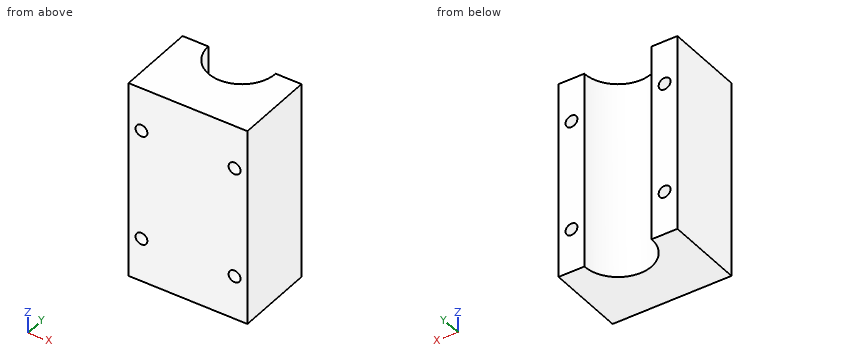
from build123d import *

# Parameters (mm, degrees)
F0_W     = 60
F0_H     = 40
F1_DEPTH = 100
F2_R     = 17
F3_DEPTH = 100
F4_R     = 3
F5_DEPTH = 45


with BuildPart() as f1:
    # F0 (on Top) → F1 (new body)
    with BuildSketch(Plane.XY):
        with Locations((0, -20)):
            Rectangle(F0_W, F0_H)
    extrude(amount=F1_DEPTH)

    # F2 (on face) → F3 (cut)
    with BuildSketch(Plane.XY.offset(100)):
        Circle(F2_R)
    extrude(amount=-F3_DEPTH, mode=Mode.SUBTRACT)

    # F4 (on face) → F5 (cut)
    with BuildSketch(Plane.XZ.offset(40)):
        with Locations((-23.5, 78)):
            Circle(F4_R)
        with Locations((-23.5, 22)):
            Circle(F4_R)
        with Locations((23.5, 22)):
            Circle(F4_R)
        with Locations((23.5, 78)):
            Circle(F4_R)
    extrude(amount=-F5_DEPTH, mode=Mode.SUBTRACT)


solid = f1.part
Could you check a few things on this model? Use its own coordinates, in mm. Give positions to 0.01 mm unless a question says otherwise; leave off trailing zeros. Order: outer loops, then holes, each group sorted by start corner. A loop starts at its lowest first (then second) coordinate and runs counter-clockwise, first axis right, second up.
Item 1: I need wall thicknesses on line 1 (Z direction, x = 23.5, y = -6); line 2 (Z direction, x = -26, y = -26.5); line 3 (X direction, y = -11.5, z = 75.5). Which ranges of each line are inside material? Lowest first, please.
Item 2: If we section it at B-B, the plane z = 78: Write out the boundary of the cut face in (x, y).
Item 3: I'm going to push flat-ended pins straight in: pin 1 (2 mm diameter, centred on x = -13, z = 10, fed in from +Y); pin 2 (9.5 mm diameter, centred on x = -23.5, z = 78, fed in from -Y); pin 3 (4 mm diameter, centred on x = -1, z = 44.5, fed in from +Y); pin 4 (12 mm diameter, centred on x = 1, z = 29.5, fed in from +Y). Where does each tip first touch, or does it pass through?
Item 4: If we section it at A-A, the plane x = 23.5: Write out the boundary of the cut face in (y, z).
Item 5: If we section it at C-C, the plane y = -4: Write out the boundary of the cut face in (x, z).
Item 6: If we section it at D-D, the plane y = -24: Write out the boundary of the cut face in (x, z), plus the area to 3 significant figures.
Values:
1. line 1: z = 0 to 19, 25 to 75, 81 to 100
1. line 2: z = 0 to 20.34, 23.66 to 76.34, 79.66 to 100
1. line 3: x = -30 to -25.16, -21.84 to -12.52, 12.52 to 21.84, 25.16 to 30
2. outline: (-30, -40) - (-26.5, -40) - (-26.5, 0) - (-30, 0) - close; (-20.5, -40) - (20.5, -40) - (20.5, 0) - (17, 0) arc R17 cw to (-17, 0) - (-20.5, 0) - close; (26.5, -40) - (30, -40) - (30, 0) - (26.5, 0) - close
3. pin 1: stops at y = -9.64
3. pin 2: stops at y = -40
3. pin 3: stops at y = -16.73
3. pin 4: stops at y = -15.49
4. outline: (-40, 0) - (0, 0) - (0, 19) - (-40, 19) - close; (-40, 25) - (0, 25) - (0, 75) - (-40, 75) - close; (-40, 81) - (0, 81) - (0, 100) - (-40, 100) - close
5. outline: (-30, 0) - (-16.52, 0) - (-16.52, 100) - (-30, 100) - close; (16.52, 0) - (30, 0) - (30, 100) - (16.52, 100) - close; hole circle Ø6 at (-23.5, 22); hole circle Ø6 at (-23.5, 78); hole circle Ø6 at (23.5, 22); hole circle Ø6 at (23.5, 78)
6. outline: (-30, 0) - (30, 0) - (30, 100) - (-30, 100) - close; hole circle Ø6 at (-23.5, 22); hole circle Ø6 at (-23.5, 78); hole circle Ø6 at (23.5, 22); hole circle Ø6 at (23.5, 78)
6. area: 5,890 mm2
